from build123d import *

# Parameters (mm, degrees)
EXTRUDE_1_DEPTH = 27.6
SKETCH_2_W      = 10
SKETCH_2_H      = 1.35
SKETCH_3_W      = 1.25
SKETCH_3_H      = 0.2


with BuildPart() as part:
    # 草图1 → 凸台-拉伸1 (new body)
    with BuildSketch(Plane.XY):
        Polygon((-3.1, 0), (3.1, 0), (3.1, 3.9), (2.5, 4.246410162), (2.5, 5.5), (-2.5, 5.5), (-2.5, 4.246410162), (-3.1, 3.9), align=None)
    extrude(amount=-EXTRUDE_1_DEPTH)

    # 草图2 → 旋转1 (revolve)
    with BuildSketch(Plane(origin=(0, 0, 0), x_dir=(0, 0, -1), z_dir=(1, 0, 0))):
        with Locations((32.6, 3.425)):
            Rectangle(SKETCH_2_W, SKETCH_2_H)
    revolve(axis=Axis((0, 2.75, -37.6), (0, 0, 1)))

    # 草图3 → 切除-旋转1 (revolve, cut)
    with BuildSketch(Plane(origin=(0, 0, 0), x_dir=(0, 0, -1), z_dir=(1, 0, 0))):
        with Locations((3.125, 5.4)):
            Rectangle(SKETCH_3_W, SKETCH_3_H)
    revolve(axis=Axis((0, 5.3, -2.5), (0, 1, 0)), mode=Mode.SUBTRACT)


solid = part.part
Could you check a few things on this model? Use its own coordinates, in mm. A direction names the side the tool comes from. Coordinates: 2 decimals unless noted, no trailing zeros. Loops run counter-clockwise (first coordinate to the right, second up) from the corner with the lowest first, then second, coordinate; pieces in that order, holes last.
1. Imagine slicing it at D-D (z = -2.5). Please give me the cut outline in (x, y).
2. We'd pull the mould along Z, two halves only. Please class faces 4 (the face through (0, 3, -37.6)), 5 (the face through (0, 5.3, -3)), 6 (the face through (2.5, 5, -14)): released by +Z, released by -Z, zero draft, split by the parting line, or undercut.
3. For P1, Ø1.5, axis at x = 0, z = -2.5, coming from the +Y side; P2, Ø1, axis at y = 2.5, z = -30, coming from the +X side, each with a flat end and sliding along its axis, tell me the tip position at first contact or that it passes through.
4. For faces 1 (the face through (0.82, 1.68, -32.67)), 2 (the face through (-3.1, 2, -14)), 3 (the face through (-2.5, 5, -14)), which set-ups out of +Z, -Z, +X, -X, +Y, -Y let a thin tool reach every point of the face, with its end or its side?
5. Imagine slicing it at A-A (x = 0). Please give me the cut outline in (y, z), and give its area (3 significant figures).
6. Imagine slicing it at C-C (y = 2.75). Please give me the cut outline in (x, z).
7. I need wall thicknesses on L1, parallel to Z at x = 0, y = 5.45; L2, parallel to X at y = 5.45, z = -2.5; L3, parallel to Z at x = 2.25, y = 0.9. Which ranges of each line are inside material? Lowest first, please.
8. Imagine slicing it at B-B (z = -17). Please give me the cut outline in (x, y), and give its area (3 significant figures).
Computed values:
1. outline: (-3.1, 0) - (3.1, 0) - (3.1, 3.9) - (2.5, 4.25) - (2.5, 5.5) - (1.25, 5.5) - (1.25, 5.3) - (-1.25, 5.3) - (-1.25, 5.5) - (-2.5, 5.5) - (-2.5, 4.25) - (-3.1, 3.9) - close
2. face 4: released by -Z
2. face 5: undercut
2. face 6: zero draft
3. P1: stops at y = 5.3
3. P2: stops at x = 1.35
4. face 1: -Z
4. face 2: +Z, -Z, -X, +Y, -Y
4. face 3: +Z, -Z, -X, +Y
5. outline: (0, -27.6) - (1.4, -27.6) - (1.4, -37.6) - (4.1, -37.6) - (4.1, -27.6) - (5.5, -27.6) - (5.5, -3.75) - (5.3, -3.75) - (5.3, -1.25) - (5.5, -1.25) - (5.5, 0) - (0, 0) - close
5. area: 178 mm2
6. outline: (-3.1, -27.6) - (-1.35, -27.6) - (-1.35, -37.6) - (1.35, -37.6) - (1.35, -27.6) - (3.1, -27.6) - (3.1, 0) - (-3.1, 0) - close
7. L1: z = -27.6 to -3.75, -1.25 to 0
7. L2: x = -2.5 to -1.25, 1.25 to 2.5
7. L3: z = -27.6 to 0
8. outline: (-3.1, 0) - (3.1, 0) - (3.1, 3.9) - (2.5, 4.25) - (2.5, 5.5) - (-2.5, 5.5) - (-2.5, 4.25) - (-3.1, 3.9) - close
8. area: 32.4 mm2
